```python
from build123d import *

# Parameters (mm, degrees)
BOSS_EXTRUDE1_DEPTH      = 50
BOSS_EXTRUDE1_DEPTH_BACK = 50
CUT_EXTRUDE1_DEPTH       = 188.082869339
CUT_EXTRUDE1_DEPTH_BACK  = 188.082869339
SKETCH2_W                = 50
SKETCH2_H                = 200
SKETCH3_R                = 37.5
BOSS_EXTRUDE2_DEPTH      = 5
CUT_EXTRUDE2_START       = -10
CUT_EXTRUDE2_DEPTH       = 10
FILLET1_R                = 10
FILLET2_R                = 4
FILLET1_OF_MIRROR2_R     = 10
FILLET2_OF_MIRROR2_R     = 4
SKETCH5_R                = 15
CUT_EXTRUDE3_DEPTH       = 10


with BuildPart() as part:
    # Sketch1 → Boss-Extrude1 (new, two sides: drawn at the far end of the back side and taken through both)
    with BuildSketch(Plane(origin=(0, 0, 0), x_dir=(0, 0, -1), z_dir=(1, 0, 0)).offset(-BOSS_EXTRUDE1_DEPTH_BACK)):
        with BuildLine():
            Line((-100, -50), (100, -50))
            ThreePointArc((100, -50), (150, 0), (100, 50))
            Line((100, 50), (-100, 50))
            ThreePointArc((-100, 50), (-150, 0), (-100, -50))
        make_face()
    extrude(amount=BOSS_EXTRUDE1_DEPTH + BOSS_EXTRUDE1_DEPTH_BACK)

    # Sketch2 → Cut-Extrude1 (cut, two sides: drawn at the far end of the back side and taken through both)
    with BuildSketch(Plane(origin=(0, 50, 0), x_dir=(1, 0, 0), z_dir=(0, 1, 0)).offset(-CUT_EXTRUDE1_DEPTH_BACK)):
        with Locations((0, 150)):
            Rectangle(SKETCH2_W, SKETCH2_H)
    extrude(amount=CUT_EXTRUDE1_DEPTH + CUT_EXTRUDE1_DEPTH_BACK, mode=Mode.SUBTRACT)

    # Sketch3 → Boss-Extrude2 (add)
    with BuildSketch(Plane(origin=(50, 0, 0), x_dir=(0, 0, -1), z_dir=(1, 0, 0))):
        with Locations(Location((100, 0, 0), (0, 0, 180))):
            Circle(SKETCH3_R)
    boss_extrude2 = extrude(amount=BOSS_EXTRUDE2_DEPTH)

    # Mirror1: Boss-Extrude2 across plane
    add(boss_extrude2.mirror(Plane(origin=(0, 0, 0), x_dir=(0, 0, 1), z_dir=(1, 0, 0))))

    # Sketch4 → Cut-Extrude2 (cut)
    with BuildSketch(Plane(origin=(50, 0, 0), x_dir=(0, 0, -1), z_dir=(1, 0, 0)).offset(CUT_EXTRUDE2_START)):
        with BuildLine():
            ThreePointArc((50.46067679, 6.77166567), (56.899460157, 25.344495759), (70, 40))
            Line((70, 40), (-70, 40))
            ThreePointArc((-70, 40), (-56.899460157, 25.344495759), (-50.46067679, 6.77166567))
            Line((-50.46067679, 6.77166567), (0, -33.596875763))
            Line((0, -33.596875763), (50.46067679, 6.77166567))
        make_face()
        with BuildLine():
            ThreePointArc((-50.373979518, -6.103940623), (-56.729785131, -25.053712404), (-70, -40))
            Line((-70, -40), (-8.003905297, -40))
            Line((-8.003905297, -40), (-50.373979518, -6.103940623))
        make_face()
        with BuildLine():
            Line((8.003905297, -40), (70, -40))
            ThreePointArc((70, -40), (56.729785131, -25.053712404), (50.373979518, -6.103940623))
            Line((50.373979518, -6.103940623), (8.003905297, -40))
        make_face()
    cut_extrude2 = extrude(amount=CUT_EXTRUDE2_DEPTH, mode=Mode.SUBTRACT)

    # Fillet1
    fillet1_edges = [part.edges().sort_by_distance(p)[0] for p in [
        (45, 6.77166567, 50.46067679),
        (45, 6.77166567, -50.46067679),
        (45, -33.596875763, 0),
    ]]
    fillet(fillet1_edges, radius=FILLET1_R)

    # Fillet2
    fillet2_edges = [part.edges().sort_by_distance(p)[0] for p in [
        (45, -6.103940623, -50.373979518),
        (45, -40, -70),
        (45, -40, -8.003905297),
        (45, -40, 70),
        (45, -6.103940623, 50.373979518),
        (45, -40, 8.003905297),
        (45, 40, 70),
        (45, 40, -70),
    ]]
    fillet(fillet2_edges, radius=FILLET2_R)

    # Mirror2: Cut-Extrude2 across plane
    add(cut_extrude2.mirror(Plane(origin=(0, 0, 0), x_dir=(0, 0, 1), z_dir=(1, 0, 0))), mode=Mode.SUBTRACT)

    # Fillet1 of Mirror2
    fillet1_of_mirror2_edges = [part.edges().sort_by_distance(p)[0] for p in [
        (-45, 6.77166567, 50.46067679),
        (-45, 6.77166567, -50.46067679),
        (-45, -33.596875763, 0),
    ]]
    fillet(fillet1_of_mirror2_edges, radius=FILLET1_OF_MIRROR2_R)

    # Fillet2 of Mirror2
    fillet2_of_mirror2_edges = [part.edges().sort_by_distance(p)[0] for p in [
        (-45, -6.103940623, -50.373979518),
        (-45, -40, -70),
        (-45, -40, -8.003905297),
        (-45, -40, 70),
        (-45, -6.103940623, 50.373979518),
        (-45, -40, 8.003905297),
        (-45, 40, 70),
        (-45, 40, -70),
    ]]
    fillet(fillet2_of_mirror2_edges, radius=FILLET2_OF_MIRROR2_R)

    # Sketch5 → Cut-Extrude3 (cut)
    with BuildSketch(Plane(origin=(55, 0, 0), x_dir=(0, 0, -1), z_dir=(1, 0, 0))):
        with Locations((100, 0)):
            Circle(SKETCH5_R)
    cut_extrude3 = extrude(amount=-CUT_EXTRUDE3_DEPTH, mode=Mode.SUBTRACT)

    # Mirror3: Cut-Extrude3 across plane
    add(cut_extrude3.mirror(Plane(origin=(0, 0, 0), x_dir=(0, 0, 1), z_dir=(1, 0, 0))), mode=Mode.SUBTRACT)


solid = part.part
```
Model file for the job. Use its own axes, mm. A direction names the side the tool comes from. Coordinates: 2 decimals unless noted, no trailing zeros. Write each loop counter-clockwise with the first axis right and the second up, starting at its lowest first coordinate (ties: lowest second). Pieces come first, ordered by that corner, then holes. Notation, with made-up numbers: (-22.75, 72) - (-5.75, 72) arc R13 ccw to (-5.75, 78) - close; hole circle Ø9 at (55, 18). An arc over 180 degrees is marked (long way). Use a Markdown table: item, result. Add a question column.
Item 1: Drill centre lines: line 1 along X through (y, z) = (19.5, -108); line 2 along X through (y, z) = (33.5, -127.5); line 3 along Y through (x, z) = (51, -100). Where is each one in solid material? Low to high.
Item 2: Two-plate mould, pull along Z, no slides. Class faces 4 (the face through (25, -1, -99)), 5 (the face through (44.93, -12.328, -26.586)), 6 (the face through (-37.675, -1.099, -149.988)): pulls with the +Z half, pulls with the -Z half, needs draft (parallel to the pull), parting line crosses it, or undercut.
Item 3: 3-axis set-ups, long thin cutter, end or side, ignore diameter. For faces 1 (the face through (37.325, -1.099, -149.988)), 2 (the face through (45.1, -9.6, -49)), 3 (the face through (-40, 13, 1)): which of +Z, -Z, +X, -X, +Y, -Y reach the whole face in a straight line?
Item 4: Drop flat-ended pins along their axis: pin 1 (24.5 mm diameter, centred on y = -30, z = -31, fed in from -X); pin 2 (15.5 mm diameter, centred on y = -26, z = -27.5, fed in from +X); pin 3 (1.5 mm diameter, centred on x = 8.5, y = -7, fed in from -Z); pin 4 (15 mm diameter, centred on y = 7, z = -93.5, fed in from +X). Give the stop position or say it passes through.
Item 5: Band-saw the part on D-D, the plane z = 37.5. Write the cut outline in (x, y), and give its area (3 significant figures).
Item 6: Band-saw the part on C-C, the plane z = -11.5. Write the cut outline in (x, y), and give its area (3 significant figures).
Item 7: Band-saw the part on A-A, the plane x = -32.5. Write the cut outline in (y, z).
A:
| question | item | result |
|---|---|---|
| 1 | line 1 | x = -55 to -25, 25 to 55 |
| 1 | line 2 | x = -50 to -25, 25 to 50 |
| 1 | line 3 | y = -37.5 to -15, 15 to 37.5 |
| 2 | face 4 | needs draft |
| 2 | face 5 | undercut |
| 2 | face 6 | pulls with the -Z half |
| 3 | face 1 | -Z, +X, -X |
| 3 | face 2 | +X |
| 3 | face 3 | -X |
| 4 | pin 1 | stops at x = -50 |
| 4 | pin 2 | stops at x = 50 |
| 4 | pin 3 | stops at z = -50 |
| 4 | pin 4 | stops at x = 55 |
| 5 | outline | (-50, -50) - (50, -50) - (50, -40) - (40, -40) - (40, -16.4) - (50, -16.4) - (50, -3.6) - (40, -3.6) - (40, 40) - (50, 40) - (50, 50) - (-50, 50) - (-50, 40) - (-40, 40) - (-40, -3.6) - (-50, -3.6) - (-50, -16.4) - (-40, -16.4) - (-40, -40) - (-50, -40) - close |
| 5 | area | 8,660 mm² |
| 6 | outline | (-50, -50) - (50, -50) - (50, -24.4) - (40, -24.4) - (40, 40) - (50, 40) - (50, 50) - (-50, 50) - (-50, 40) - (-40, 40) - (-40, -24.4) - (-50, -24.4) - close |
| 6 | area | 8,710 mm² |
| 7 | outline | (-50, -100) arc R50 ccw to (50, -100) - (50, 100) arc R50 ccw to (-50, 100) - close |
